from build123d import *

# Parameters (mm, degrees)
SKETCH_1_W          = 80
SKETCH_1_H          = 120
EXTRUDE_1_DEPTH     = 6
SKETCH_2_W          = 80
SKETCH_2_H          = 6
EXTRUDE_2_DEPTH     = 50
FILLET_1_R          = 4
FILLET_2_R          = 10
CUT_EXTRUDE_1_REACH = 8
SKETCH_3_R          = 5
EXTRUDE_3_DEPTH     = 3
SKETCH_5_R          = 4
CUT_EXTRUDE_2_DEPTH = 6
FILLET_3_R          = 20


with BuildPart() as part:
    # 草图1 → 凸台-拉伸1 (new body)
    with BuildSketch(Plane.XY):
        with Locations((40, 60)):
            Rectangle(SKETCH_1_W, SKETCH_1_H)
    extrude(amount=EXTRUDE_1_DEPTH)

    # 草图2 → 凸台-拉伸2 (add)
    with BuildSketch(Plane.XY.offset(6)):
        with Locations((40, 3)):
            Rectangle(SKETCH_2_W, SKETCH_2_H)
    extrude(amount=EXTRUDE_2_DEPTH)

    # 圆角1
    fillet_1_edges = [part.edges().sort_by_distance(p)[0] for p in [
        (40, 6, 6),
    ]]
    fillet(fillet_1_edges, radius=FILLET_1_R)

    # 圆角2
    fillet_2_edges = [part.edges().sort_by_distance(p)[0] for p in [
        (40, 0, 0),
    ]]
    fillet(fillet_2_edges, radius=FILLET_2_R)

    # 草图3 → 切除-拉伸1 (cut, up to next)
    with BuildSketch(Plane.XY.offset(6), mode=Mode.PRIVATE) as cut_extrude_1_sk1:
        with Locations((60, 105)):
            Circle(SKETCH_3_R)
    cut_extrude_1_tool1 = extrude(cut_extrude_1_sk1.sketch, amount=-CUT_EXTRUDE_1_REACH, mode=Mode.PRIVATE) & part.part
    add(cut_extrude_1_tool1.solids().sort_by_distance((60, 105, 6))[0], mode=Mode.SUBTRACT)
    # 草图3 → 切除-拉伸1 (cut, up to next)
    with BuildSketch(Plane.XY.offset(6), mode=Mode.PRIVATE) as cut_extrude_1_sk2:
        with Locations((20, 105)):
            Circle(SKETCH_3_R)
    cut_extrude_1_tool2 = extrude(cut_extrude_1_sk2.sketch, amount=-CUT_EXTRUDE_1_REACH, mode=Mode.PRIVATE) & part.part
    add(cut_extrude_1_tool2.solids().sort_by_distance((20, 105, 6))[0], mode=Mode.SUBTRACT)
    # 草图3 → 切除-拉伸1 (cut, up to next)
    with BuildSketch(Plane.XY.offset(6), mode=Mode.PRIVATE) as cut_extrude_1_sk3:
        with Locations((20, 25)):
            Circle(SKETCH_3_R)
    cut_extrude_1_tool3 = extrude(cut_extrude_1_sk3.sketch, amount=-CUT_EXTRUDE_1_REACH, mode=Mode.PRIVATE) & part.part
    add(cut_extrude_1_tool3.solids().sort_by_distance((20, 25, 6))[0], mode=Mode.SUBTRACT)
    # 草图3 → 切除-拉伸1 (cut, up to next)
    with BuildSketch(Plane.XY.offset(6), mode=Mode.PRIVATE) as cut_extrude_1_sk4:
        with Locations((60, 25)):
            Circle(SKETCH_3_R)
    cut_extrude_1_tool4 = extrude(cut_extrude_1_sk4.sketch, amount=-CUT_EXTRUDE_1_REACH, mode=Mode.PRIVATE) & part.part
    add(cut_extrude_1_tool4.solids().sort_by_distance((60, 25, 6))[0], mode=Mode.SUBTRACT)

    # 草图4 → 凸台-拉伸3 (add, symmetric)
    with BuildSketch(Plane(origin=(40, 0, 0), x_dir=(0, 0, -1), z_dir=(1, 0, 0))):
        Polygon((-51, 6), (-10, 6), (-6, 10), (-6, 116), (-11, 116), (-51, 11), align=None)
    extrude(amount=EXTRUDE_3_DEPTH, both=True)

    # 草图5 → 切除-拉伸2 (cut)
    with BuildSketch(Plane(origin=(0, 6, 0), x_dir=(1, 0, 0), z_dir=(0, 1, 0))):
        with Locations((25, -31)):
            Circle(SKETCH_5_R)
        with Locations((55, -31)):
            Circle(SKETCH_5_R)
    extrude(amount=-CUT_EXTRUDE_2_DEPTH, mode=Mode.SUBTRACT)

    # 圆角3
    fillet_3_edges = [part.edges().sort_by_distance(p)[0] for p in [
        (0, 3, 56),
        (80, 3, 56),
    ]]
    fillet(fillet_3_edges, radius=FILLET_3_R)


solid = part.part
Input: part model. Units: mm. Frame: model coordinates. A direction names the side the tool comes from. Give positions to 0.01 mm unless a question says otherwise; leave off trailing zeros. Order: outer loops, then holes, each group sorted by start corner. A loop starts at its lowest first (then second) coordinate and runs counter-clockwise, first axis right, second up. Notation, with made-up numbers: M 83.5,-34 L 92.5,-34 A8 ccw 92.5,-21 Z; hole C 5,50.25 d4. An arc over 180 degrees is marked long. Answer as a JSON object with one key per item and string values.
1. Cut plane D-D, the plane z = 32.5. Output: boundary loops of the cut face in (x, y).
Result sheet:
{"outline": "M 0,0 L 21.29,0 L 21.29,6 L 0,6 Z; M 28.71,0 L 51.29,0 L 51.29,6 L 43,6 L 43,59.56 L 37,59.56 L 37,6 L 28.71,6 Z; M 58.71,0 L 80,0 L 80,6 L 58.71,6 Z"}
2. Reachability of faces 1 (the cylindrical face through (18.92, 100.12, 3.04)), 2 (the flat face through (40, 116, 8)), 3 (the flat face through (37, 50, 24)) from +Z, -Z, +X, -X, +Y, -Y: full face, straight path, thin tool, end or side. Return the list, or none.
Result sheet:
{"face 1": "+Z, -Z", "face 2": "+Z, +X, -X, +Y", "face 3": "+Z, -X, +Y"}
3. Cut plane B-B, the plane y = 105. Output: boundary loops of the cut face in (x, z), and give its area (3 significant figures).
Result sheet:
{"outline": "M 0,0 L 15,0 L 15,6 L 0,6 Z; M 25,0 L 55,0 L 55,6 L 43,6 L 43,15.19 L 37,15.19 L 37,6 L 25,6 Z; M 65,0 L 80,0 L 80,6 L 65,6 Z", "area": "415 mm²"}
4. Ray query, line 1 (Y direction, x = 20, z = 2.3); line 2 (Y direction, x = 60, z = 3.5); line 3 (Z direction, x = 12, y = 52.5). Return the intervals inside material, ascending. Write a range as [from, to].
Result sheet:
{"line 1": "[3.62, 20], [30, 100], [110, 120]", "line 2": "[2.4, 20], [30, 100], [110, 120]", "line 3": "[0, 6]"}
5. First-contact query: P1, Ø1, axis at x = 66.5, y = 95.5, coming from the +Z side; P2, Ø8, axis at x = 60, y = 25, coming from the +Z side; P3, Ø1, axis at y = 24, z = 24.5, coming from the +X side; P4, Ø22.5, axis at y = 70.5, z = 28, coming from the -X side. Flat tips, straight axial feed; report the tip coordinate or a pass-through.
Result sheet:
{"P1": "z = 6", "P2": "through", "P3": "x = 43", "P4": "x = 37"}
6. Cut plane A-A, the plane z = 7.5. Output: boundary loops of the cut face in (x, y), and give its area (3 significant figures).
Result sheet:
{"outline": "M 0,0.32 L 80,0.32 L 80,6.88 L 0,6.88 Z; M 37,8.5 L 43,8.5 L 43,116 L 37,116 Z", "area": "1,170 mm²"}
7. Pull-direction query (X, two-part tool) for faces 4 (the cylindrical face through (5.703, 3.042, 49.986)), 5 (the flat face through (39, 66, 0)), 6 (the cylindrical face through (58.92, 20.12, 3.04)), 7 (the cylindrical face through (24.479, 3.042, 27.034)); classes: +X half, -X half, draft (parallel to the pull), parting line (faces both ways), or undercut.
Result sheet:
{"face 4": "-X half", "face 5": "draft", "face 6": "undercut", "face 7": "undercut"}
8. Cut plane C-C, the plane x = 46.5. Output: boundary loops of the cut face in (y, z).
Result sheet:
{"outline": "M 0,10 A10 ccw 10,0 L 120,0 L 120,6 L 10,6 A4 cw 6,10 L 6,56 L 0,56 Z"}
